Design review of the part built by this model. Coordinates are the model's own, in mm. A direction names the side the tool comes from. Coordinates: 2 decimals unless noted, no trailing zeros. Write each loop counter-clockwise with the first axis right and the second up, starting at its lowest first coordinate (ties: lowest second). Pieces come first, ordered by that corner, then holes. Notation, with made-up numbers: M -16.75,51 L 31.25,51 A27 cw 31.25,80 Z; hole C 19,-37 d9. An arc over 180 degrees is marked long. Write item = value, one per line.
```python
from build123d import *

# Parameters (mm, degrees)
SKETCH1_W                = 90
SKETCH1_H                = 30
BOSS_EXTRUDE1_DEPTH      = 4
FILLET1_R                = 10
SKETCH2_R                = 1.25
CUT_EXTRUDE1_DEPTH       = 48.602520942
SKETCH3_R                = 1.25
CUT_EXTRUDE2_DEPTH       = 48.602520942
SKETCH4_W                = 16
SKETCH4_H                = 30
BOSS_EXTRUDE5_DEPTH      = 3
SKETCH11_W               = 3
SKETCH11_H               = 30
BOSS_EXTRUDE6_DEPTH      = 39
SKETCH12_W               = 16
SKETCH12_H               = 30
BOSS_EXTRUDE7_DEPTH      = 3
SKETCH14_R               = 1.575
CUT_EXTRUDE7_DEPTH       = 3
SKETCH13_R               = 1.575
CUT_EXTRUDE8_DEPTH       = 3
FILLET2_R                = 5
CUT_EXTRUDE10_START      = -30
CUT_EXTRUDE10_DEPTH      = 30
CUT_EXTRUDE11_DEPTH      = 73.97944927
CUT_EXTRUDE11_DEPTH_BACK = 73.97944927
FILLET3_R                = 1
SKETCH18_R               = 11
CUT_EXTRUDE12_DEPTH      = 2
SKETCH19_R               = 11
CUT_EXTRUDE13_DEPTH      = 2
SKETCH20_R               = 5.25
CUT_EXTRUDE14_DEPTH      = 2
SKETCH21_R               = 5.25
CUT_EXTRUDE15_DEPTH      = 2


# Read off the part's stored shape, not the designer's step: Cut-Extrude10
with BuildPart() as part:
    # Sketch1 → Boss-Extrude1 (new body)
    with BuildSketch(Plane(origin=(0, 0, 0), x_dir=(0, 0, -1), z_dir=(1, 0, 0))):
        Rectangle(SKETCH1_W, SKETCH1_H)
    extrude(amount=BOSS_EXTRUDE1_DEPTH)

    # Fillet1
    fillet1_edges = [part.edges().sort_by_distance(p)[0] for p in [
        (2, -15, -45),
        (2, -15, 45),
        (2, 15, 45),
        (2, 15, -45),
    ]]
    fillet(fillet1_edges, radius=FILLET1_R)

    # Sketch2 → Cut-Extrude1 (cut, through all)
    with BuildSketch(Plane(origin=(4, 0, 0), x_dir=(0, 0, -1), z_dir=(1, 0, 0))):
        with Locations((-30, 0)):
            Circle(SKETCH2_R)
    extrude(amount=-CUT_EXTRUDE1_DEPTH, mode=Mode.SUBTRACT)

    # Sketch3 → Cut-Extrude2 (cut, through all)
    with BuildSketch(Plane(origin=(4, 0, 0), x_dir=(0, 0, -1), z_dir=(1, 0, 0))):
        with Locations((30, 0)):
            Circle(SKETCH3_R)
    extrude(amount=-CUT_EXTRUDE2_DEPTH, mode=Mode.SUBTRACT)

    # Sketch4 → Boss-Extrude5 (add)
    with BuildSketch(Plane(origin=(4, 0, 0), x_dir=(0, 0, -1), z_dir=(1, 0, 0))):
        Rectangle(SKETCH4_W, SKETCH4_H)
    extrude(amount=BOSS_EXTRUDE5_DEPTH)

    # Sketch11 → Boss-Extrude6 (add)
    with BuildSketch(Plane(origin=(7, 0, 0), x_dir=(0, 0, -1), z_dir=(1, 0, 0))):
        Rectangle(SKETCH11_W, SKETCH11_H)
    extrude(amount=BOSS_EXTRUDE6_DEPTH)

    # Sketch12 → Boss-Extrude7 (add)
    with BuildSketch(Plane(origin=(46, 0, 0), x_dir=(0, 0, -1), z_dir=(1, 0, 0))):
        Rectangle(SKETCH12_W, SKETCH12_H)
    extrude(amount=BOSS_EXTRUDE7_DEPTH)

    # Sketch14 → Cut-Extrude7 (cut)
    with BuildSketch(Plane(origin=(49, 0, 0), x_dir=(0, 0, -1), z_dir=(1, 0, 0))):
        with Locations((4.75, 0)):
            Circle(SKETCH14_R)
    extrude(amount=-CUT_EXTRUDE7_DEPTH, mode=Mode.SUBTRACT)

    # Sketch13 → Cut-Extrude8 (cut)
    with BuildSketch(Plane(origin=(49, 0, 0), x_dir=(0, 0, -1), z_dir=(1, 0, 0))):
        with Locations((-4.75, 0)):
            Circle(SKETCH13_R)
    extrude(amount=-CUT_EXTRUDE8_DEPTH, mode=Mode.SUBTRACT)

    # Fillet2
    fillet2_edges = [part.edges().sort_by_distance(p)[0] for p in [
        (7, 0, -1.5),
        (7, 0, 1.5),
    ]]
    fillet(fillet2_edges, radius=FILLET2_R)

    # Cut-Extrude10 outline → Cut-Extrude10 (cut)
    with BuildSketch(Plane.XZ.offset(15).offset(CUT_EXTRUDE10_START)):
        with BuildLine():
            add(Edge.make_bspline(
                [(12, 1.5), (8.564078645, 1.5), (4, 3.226164853), (4, 8)],
                knots=[0, 0, 0, 0, 1, 1, 1, 1], degree=3))
            ThreePointArc((12, 1.5), (8.464466094, 2.964466094), (7, 6.5))
            Line((7, 6.5), (7, 8))
            Line((7, 8), (4, 8))
        make_face()
    extrude(amount=CUT_EXTRUDE10_DEPTH, mode=Mode.SUBTRACT)

    # Sketch16 → Cut-Extrude11 (cut, two sides: drawn at the far end of the back side and taken through both)
    with BuildSketch(Plane.XZ.offset(15).offset(-CUT_EXTRUDE11_DEPTH_BACK)):
        with BuildLine():
            ThreePointArc((7, -6.5), (8.464466094, -2.964466094), (12, -1.5))
            add(Edge.make_bspline(
                [(12, -1.5), (8.564078645, -1.5), (4, -3.006580432), (4, -8)],
                knots=[0, 0, 0, 0, 1, 1, 1, 1], degree=3))
            Line((4, -8), (7, -8))
            Line((7, -8), (7, -6.5))
        make_face()
    extrude(amount=CUT_EXTRUDE11_DEPTH + CUT_EXTRUDE11_DEPTH_BACK, mode=Mode.SUBTRACT)

    # Fillet3
    fillet3_edges = [part.edges().sort_by_distance(p)[0] for p in [
        (46, 0, -1.5),
        (46, 0, 1.5),
        (46, 0, 8),
        (46, 0, -8),
    ]]
    fillet(fillet3_edges, radius=FILLET3_R)

    # Sketch18 → Cut-Extrude12 (cut)
    with BuildSketch(Plane.ZY):
        with Locations((30, 0)):
            Circle(SKETCH18_R)
    extrude(amount=-CUT_EXTRUDE12_DEPTH, mode=Mode.SUBTRACT)

    # Sketch19 → Cut-Extrude13 (cut)
    with BuildSketch(Plane.ZY):
        with Locations((-30, 0)):
            Circle(SKETCH19_R)
    extrude(amount=-CUT_EXTRUDE13_DEPTH, mode=Mode.SUBTRACT)

    # Sketch20 → Cut-Extrude14 (cut)
    with BuildSketch(Plane.ZY.offset(-2)):
        with Locations((30, 0)):
            Circle(SKETCH20_R)
    extrude(amount=-CUT_EXTRUDE14_DEPTH, mode=Mode.SUBTRACT)

    # Sketch21 → Cut-Extrude15 (cut)
    with BuildSketch(Plane.ZY.offset(-2)):
        with Locations((-30, 0)):
            Circle(SKETCH21_R)
    extrude(amount=-CUT_EXTRUDE15_DEPTH, mode=Mode.SUBTRACT)


solid = part.part
```
Q1. Consider section A-A, the plane z = 30. State the section outline as (x, y) points.
Check result:
outline = M 0,-15 L 4,-15 L 4,-5.25 L 2,-5.25 L 2,-11 L 0,-11 Z; M 0,11 L 2,11 L 2,5.25 L 4,5.25 L 4,15 L 0,15 Z
Q2. Machinability: for faces 1 (the flat face through (4, 0, 23)), 2 (the flat face through (4, 0, -22)), 3 (the cylindrical face through (47.521, 0.069, -3.177)), which of the approach directions +Z, -Z, +X, -X, +Y, -Y give a long, thin tool a straight path to every point of the face, cutting with its end or side? Answer none if there is none.
Check result:
face_1 = +Z, +X, +Y, -Y
face_2 = -Z, +X, +Y, -Y
face_3 = +X
Q3. The part is to be moulded in two halves that separate along X. For faces 4 (the flat face through (28, 0, -1.5)), 5 (the flat face through (2, 0, -45)), 6 (the flat face through (2, -5, 27)), say which applies: +X half, -X half, draft (parallel to the pull), parting line (faces both ways), or undercut.
Check result:
face_4 = undercut
face_5 = draft
face_6 = -X half
Q4. Consider section D-D, the plane z = 16. State the section outline as (x, y) points, and give its area (3 significant figures).
Check result:
outline = M 0,-15 L 4,-15 L 4,15 L 0,15 Z
area = 120 mm²
Q5. For P1, Ø15, axis at y = -4, z = 34.5, coming from the +X side; P2, Ø6, axis at y = -1, z = 24, coming from the -X side; P3, Ø0.6, axis at x = 48, y = -6, coming from the -Z side; P4, Ø9.5, axis at y = 0, z = 30, coming from the +X side, all flat-tipped, find the tip position at first contact; note any pin that passes through.
Check result:
P1 = 4
P2 = 2
P3 = -8
P4 = through
Q6. Consider section C-C, the plane x = 14. State the section outline as (y, z) points, and give its area (3 significant figures).
Check result:
outline = M -15,-1.5 L 15,-1.5 L 15,1.5 L -15,1.5 Z
area = 90.0 mm²
Q7. Consider section B-B, the plane y = 0. State how many separate pieces and enclosed holes the cut face has, and give its area (3 significant figures).
Check result:
separate_pieces = 5
enclosed_holes = 0
area = 405 mm²
Q8. Wall thickness on line 1 (Y direction, x = 3, z = -30); line 2 (Z direction, x = 21, y = -9); line 3 (Y direction, x = 1.55, z = 30): over which ranges is each line inside the solid? List them lowest first.
Check result:
line_1 = -15 to -5.25, 5.25 to 15
line_2 = -1.5 to 1.5
line_3 = -15 to -11, 11 to 15
